Answer from the drawing. Dimensions are ordinates in mm from the lowest x, y and z of the part. Give positions to 0.01 mm unless a question says otherwise; leave off trailing zeros. Order: outer loops, then holes, each group sorted by start corner. A loop starts at its lowest first (then second) coordinate and runs counter-clockwise, first axis right, second up. Notation, with made-up numbers: (-9, -23.5) - (50, -23.5) arc R28 cw to (50, 0.5) - close; hole circle Ø8 at (-8.75, 29.5). An arc over 180 degrees is marked (long way). Answer in a Markdown table with one row per item.
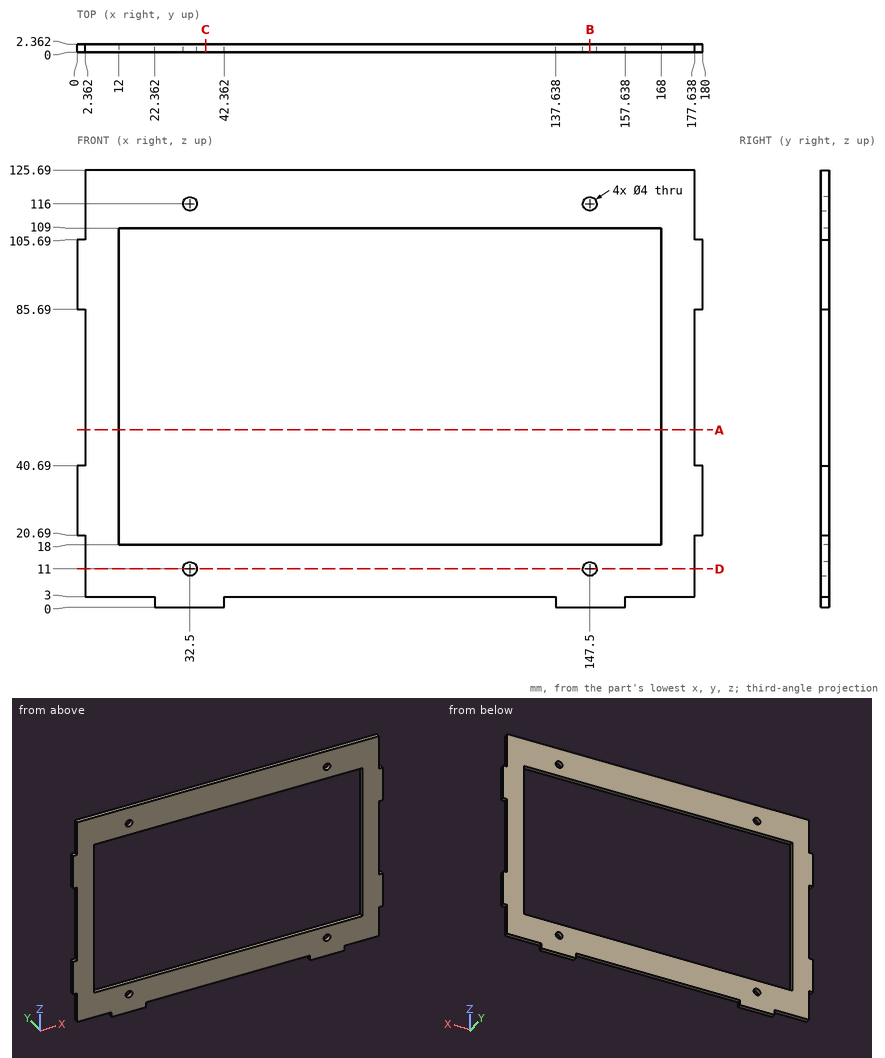
Item 1: Find section D-D on z = 11. Write down the section's boundary in (x, y), then the cut area to 3 significant figures.
Answer block:
| item | result |
|---|---|
| outline | (2.36, 0) - (30.5, 0) - (30.5, 2.36) - (2.36, 2.36) - close; (34.5, 0) - (145.5, 0) - (145.5, 2.36) - (34.5, 2.36) - close; (149.5, 0) - (177.64, 0) - (177.64, 2.36) - (149.5, 2.36) - close |
| area | 395 mm² |
Item 2: Find section B-B on x = 147.5. Write down the section's boundary in (y, z).
Answer block:
| item | result |
|---|---|
| outline | (0, 0) - (2.36, 0) - (2.36, 9) - (0, 9) - close; (0, 13) - (2.36, 13) - (2.36, 18) - (0, 18) - close; (0, 109) - (2.36, 109) - (2.36, 114) - (0, 114) - close; (0, 118) - (2.36, 118) - (2.36, 125.69) - (0, 125.69) - close |
Item 3: Consider line 1 (X direction, y = 1.8, z = 116); line 2 (Z direction, x = 147.5, y = 0.85); line 3 (Z direction, x = 86, y = 0.2). Determine where each line is inside the solid, lowest interval first.
Answer block:
| item | result |
|---|---|
| line 1 | 2.36 to 30.5, 34.5 to 145.5, 149.5 to 177.64 |
| line 2 | 0 to 9, 13 to 18, 109 to 114, 118 to 125.69 |
| line 3 | 3 to 18, 109 to 125.69 |
Item 4: Find section A-A on z = 51. Write down the section's boundary in (x, y).
Answer block:
| item | result |
|---|---|
| outline | (2.36, 0) - (12, 0) - (12, 2.36) - (2.36, 2.36) - close; (168, 0) - (177.64, 0) - (177.64, 2.36) - (168, 2.36) - close |
Item 5: Find section C-C on x = 37. Write down the section's boundary in (y, z).
Answer block:
| item | result |
|---|---|
| outline | (0, 0) - (2.36, 0) - (2.36, 18) - (0, 18) - close; (0, 109) - (2.36, 109) - (2.36, 125.69) - (0, 125.69) - close |
Item 6: Each of these flat-tipped pins is pushed along its axis until it touches: P1, Ø2.5, axis at x = 147.5, z = 11, coming from the -Y side; P2, Ø1.2, axis at y = 1, z = 1.5, coming from the -X side; P3, Ø1.2, axis at x = 87, y = 1, coming from the -Z side; P4, Ø1.2, axis at y = 1.5, z = 1.5, coming from the +X side. Where does it stop, or does it pass through?
Answer block:
| item | result |
|---|---|
| P1 | through |
| P2 | x = 22.36 |
| P3 | z = 3 |
| P4 | x = 157.64 |
